```python
from build123d import *

# Parameters (mm, degrees)
SKETCH2_W               = 99.06
SKETCH2_H               = 59.69
BOSS_EXTRUDE1_DEPTH     = 3.81
CUT_EXTRUDE1_DEPTH      = 58.952230544
CUT_EXTRUDE1_DEPTH_BACK = 58.952230544
SKETCH3_R               = 1.905
SKETCH4_W               = 66.005411874
SKETCH4_H               = 23.84908854
BOSS_EXTRUDE2_DEPTH     = 30.226


with BuildPart() as part:
    # Sketch2 → Boss-Extrude1 (new body)
    with BuildSketch(Plane(origin=(0, 0, 0), x_dir=(1, 0, 0), z_dir=(0, 1, 0))):
        Rectangle(SKETCH2_W, SKETCH2_H)
    extrude(amount=BOSS_EXTRUDE1_DEPTH)

    # Sketch3 → Cut-Extrude1 (cut, two sides: drawn at the far end of the back side and taken through both)
    with BuildSketch(Plane(origin=(0, 3.81, 0), x_dir=(1, 0, 0), z_dir=(0, 1, 0)).offset(-CUT_EXTRUDE1_DEPTH_BACK)):
        with Locations(Location((-46.99, 26.9875, 0), (0, 0, 270))):
            Circle(SKETCH3_R)
        with Locations(Location((46.99, 26.9875, 0), (0, 0, 270))):
            Circle(SKETCH3_R)
        with Locations(Location((46.99, -26.9875, 0), (0, 0, 270))):
            Circle(SKETCH3_R)
        with Locations(Location((-46.99, -26.9875, 0), (0, 0, 270))):
            Circle(SKETCH3_R)
    extrude(amount=CUT_EXTRUDE1_DEPTH + CUT_EXTRUDE1_DEPTH_BACK, mode=Mode.SUBTRACT)

    # Sketch4 → Boss-Extrude2 (add)
    with BuildSketch(Plane(origin=(0, 3.81, 0), x_dir=(1, 0, 0), z_dir=(0, 1, 0))):
        with Locations((9.522918202, -17.92045573)):
            Rectangle(SKETCH4_W, SKETCH4_H)
    extrude(amount=BOSS_EXTRUDE2_DEPTH)


solid = part.part
```
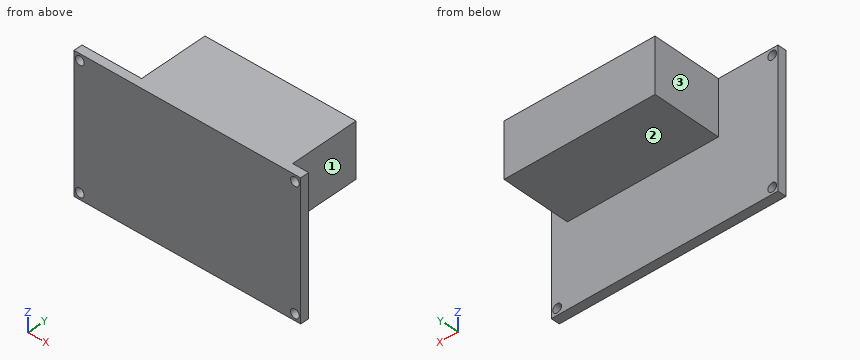
CAD build for the part. Positions are in the model's coordinates, mm. Face numbers are marked on the shaded views. A direction names the side the tool comes from. Round coordinates to 2 decimals unless told otherwise and drop trailing zeros. Loops run counter-clockwise (first coordinate to the right, second up) from the corner with the lowest first, then second, coordinate; pieces in that order, holes last. Notation, with made-up numbers: M 45.25,-17.5 L 60.25,-17.5 A7 cw 60.25,-9.5 Z; hole C 51,-2.75 d2. An arc over 180 degrees is marked long. Use a Markdown table: item, result. Add a question column.
(1) Cut at C-C (z = 26.5). Give the cut face in (x, y), and give its area (3 significant figures).
(2) Cut at A-A (x = -46.99). Give the cut face in (y, z) (1 decimal).
(3) Flat gauge pins, fed straight in: pin 1 (9 mm diameter, centred on x = 19, y = 13, fed in from -Z); pin 2 (8 mm diameter, centred on y = 12, z = 6, fed in from +X); pin 3 (2 mm diameter, centred on y = 5, z = -22.5, fed in from +X); pin 4 (12 mm diameter, centred on y = 24.5, z = 20.5, fed in from -X). Where does each tip first touch, or does it go through?
(4) Drill centre lines: line 1 (Z direction, x = -46.99, y = 2.4) (1 decimal); line 2 (Z direction, x = 40, y = 23) (3 decimals); line 3 (Y direction, x = -29, z = -19). Where is each one in solid material? Low to high.
(5) Cut at B-B (z = 7). Give the cut face in (x, y), and give its area (3 significant figures).
(6) Cut at D-D (x = 14). Give the cut face in (y, z) (3 decimals).
(7) Which spindle directions (+Z, -Z, +X, -X, +Y, -Y) get a long thin tool onto all of the face, cutting with end or side? Do the marked faces 1, 2 and 3. Say none if no direction does.
Geometry says:
| question | item | result |
|---|---|---|
| 1 | outline | M -49.53,0 L -48.83,0 L -48.83,3.81 L -49.53,3.81 Z; M -45.15,0 L 45.15,0 L 45.15,3.81 L 42.53,3.81 L 42.53,34.04 L -23.48,34.04 L -23.48,3.81 L -45.15,3.81 Z; M 48.83,0 L 49.53,0 L 49.53,3.81 L 48.83,3.81 Z |
| 1 | area | 2,340 mm² |
| 2 | outline | M 0,-29.8 L 3.8,-29.8 L 3.8,-28.9 L 0,-28.9 Z; M 0,-25.1 L 3.8,-25.1 L 3.8,25.1 L 0,25.1 Z; M 0,28.9 L 3.8,28.9 L 3.8,29.8 L 0,29.8 Z |
| 3 | pin 1 | stops at z = 6 |
| 3 | pin 2 | stops at x = 42.53 |
| 3 | pin 3 | passes through |
| 3 | pin 4 | stops at x = -23.48 |
| 4 | line 1 | z = -29.8 to -28.9, -25.1 to 25.1, 28.9 to 29.8 |
| 4 | line 2 | z = 5.996 to 29.845 |
| 4 | line 3 | y = 0 to 3.81 |
| 5 | outline | M -49.53,0 L 49.53,0 L 49.53,3.81 L 42.53,3.81 L 42.53,34.04 L -23.48,34.04 L -23.48,3.81 L -49.53,3.81 Z |
| 5 | area | 2,370 mm² |
| 6 | outline | M 0,-29.845 L 3.81,-29.845 L 3.81,5.996 L 34.036,5.996 L 34.036,29.845 L 0,29.845 Z |
| 7 | face 1 | +Z, -Z, +X, +Y |
| 7 | face 2 | -Z, +X, -X, +Y |
| 7 | face 3 | +Z, -Z, -X, +Y |
